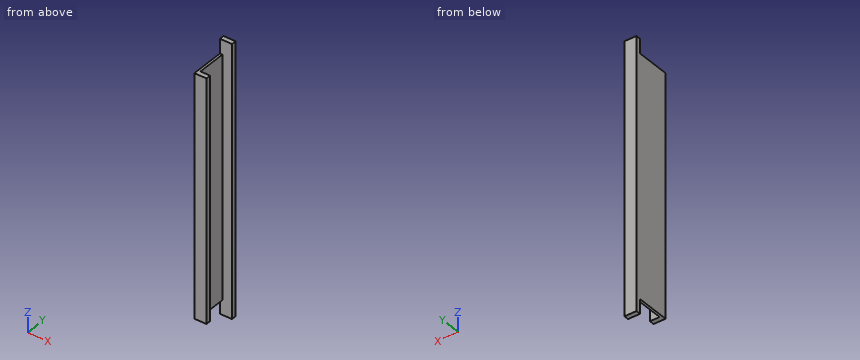
from build123d import *

# Parameters (mm, degrees)
CROQUIS1_R                   = 2.5
SALIENTE_EXTRUIR1_DEPTH      = 1.25
SALIENTE_EXTRUIR4_DEPTH      = 2.5
CROQUIS6_R                   = 12.525
CORTAR_EXTRUIR3_DEPTH        = 10
SALIENTE_EXTRUIR5_DEPTH      = 200
CROQUIS8_R                   = 12.525
SALIENTE_EXTRUIR6_DEPTH      = 21
CROQUIS10_W                  = 18.5
CROQUIS10_H                  = 25.138120499
CROQUIS10_W_2                = 2.5
CROQUIS10_H_2                = 4.861879501
CROQUIS10_H_3                = 5
CORTAR_EXTRUIR5_DEPTH        = 98
SALIENTE_EXTRUIR7_DEPTH      = 50
SALIENTE_EXTRUIR8_DEPTH      = 15
SALIENTE_EXTRUIR8_DEPTH_BACK = 265
CROQUIS15_W                  = 250
CROQUIS15_H                  = 5
CROQUIS15_W_2                = 280
SALIENTE_EXTRUIR9_DEPTH      = 7.5


with BuildPart() as part:
    # Croquis1 → Saliente-Extruir1 (new, symmetric)
    with BuildSketch(Plane(origin=(0, 0, 0), x_dir=(0, 0, -1), z_dir=(1, 0, 0))):
        with BuildLine():
            Line((125, -2.5), (-125, -2.5))
            Line((-125, -2.5), (-125, 2.5))
            Line((-125, 2.5), (-123, 2.5))
            Line((-123, 2.5), (-117, 17.5))
            ThreePointArc((-117, 17.5), (-110, 24.5), (-103, 17.5))
            Line((-103, 17.5), (-97, 2.5))
            Line((-97, 2.5), (125, 2.5))
            Line((125, 2.5), (125, -2.5))
        make_face()
        with Locations((-110, 17.5)):
            Circle(CROQUIS1_R, mode=Mode.SUBTRACT)
    extrude(amount=SALIENTE_EXTRUIR1_DEPTH, both=True)

    # Croquis5 → Saliente-Extruir4 (add, through all)
    with BuildSketch(Plane(origin=(1.25, 0, 0), x_dir=(0, 0, -1), z_dir=(1, 0, 0))):
        with BuildLine():
            ThreePointArc((-100, 10), (-110, 5), (-120, 10))
            Line((-120, 10), (-121.0552482, 7.361879501))
            ThreePointArc((-121.0552482, 7.361879501), (-110, 2.5), (-98.9447518, 7.361879501))
            Line((-98.9447518, 7.361879501), (-100, 10))
        make_face()
        with BuildLine():
            Line((-121.0552482, 7.361879501), (-120, 10))
            ThreePointArc((-120, 10), (-113.952847075, 29.358541226), (-97.5, 17.5))
            ThreePointArc((-97.5, 17.5), (-98.141458774, 13.547152925), (-100, 10))
            Line((-100, 10), (-98.9447518, 7.361879501))
            ThreePointArc((-98.9447518, 7.361879501), (-96.020931308, 12.060731804), (-95, 17.5))
            ThreePointArc((-95, 17.5), (-115.439268196, 31.479068692), (-121.0552482, 7.361879501))
        make_face()
    extrude(amount=-SALIENTE_EXTRUIR4_DEPTH)

    # Croquis6 → Cortar-Extruir3 (cut)
    with BuildSketch(Plane(origin=(1.25, 0, 0), x_dir=(0, 0, -1), z_dir=(1, 0, 0))):
        with Locations((-110, 17.5)):
            Circle(CROQUIS6_R)
    extrude(amount=-CORTAR_EXTRUIR3_DEPTH, mode=Mode.SUBTRACT)

    # Croquis7 → Saliente-Extruir5 (add)
    with BuildSketch(Plane(origin=(0, 0, -125), x_dir=(-1, 0, 0), z_dir=(0, 0, -1))):
        Polygon((3.75, 37.8), (3.75, -2.5), (1.25, -2.5), (1.25, 2.5), (1.25, 32.8), (-1.25, 32.8), (-1.25, 37.8), align=None)
    extrude(amount=-SALIENTE_EXTRUIR5_DEPTH)

    # Croquis8 → Saliente-Extruir6 (add)
    with BuildSketch(Plane.ZY.offset(1.25)):
        with BuildLine():
            Line((98.9447518, 7.361879501), (97, 2.5))
            Line((97, 2.5), (95, 2.5))
            Line((95, 2.5), (95, -2.5))
            Line((95, -2.5), (125, -2.5))
            Line((125, -2.5), (125, 2.5))
            Line((125, 2.5), (123, 2.5))
            Line((123, 2.5), (121.0552482, 7.361879501))
            ThreePointArc((121.0552482, 7.361879501), (110, 32.5), (98.9447518, 7.361879501))
        make_face()
        with Locations(Location((110, 17.5, 0), (0, 0, 180))):
            Circle(CROQUIS8_R, mode=Mode.SUBTRACT)
    extrude(amount=SALIENTE_EXTRUIR6_DEPTH)

    # Croquis10 → Cortar-Extruir5 (cut)
    with BuildSketch(Plane.XY.offset(75)):
        with Locations((-13, 19.930939751)):
            Rectangle(CROQUIS10_W, CROQUIS10_H)
        Polygon((1.25, 37.8), (-3.75, 37.8), (-3.75, 32.5), (-1.25, 32.5), (-1.25, 32.8), (1.25, 32.8), align=None)
        with Locations((0, 19.930939751)):
            Rectangle(CROQUIS10_W_2, CROQUIS10_H)
        with Locations((-2.5, 19.930939751)):
            Rectangle(CROQUIS10_W_2, CROQUIS10_H)
        with Locations((-13, 4.930939751)):
            Rectangle(CROQUIS10_W, CROQUIS10_H_2)
        with Locations((-2.5, 4.930939751)):
            Rectangle(CROQUIS10_W_2, CROQUIS10_H_2)
        with Locations((0, 4.930939751)):
            Rectangle(CROQUIS10_W_2, CROQUIS10_H_2)
        with Locations((-2.5, 0)):
            Rectangle(CROQUIS10_W_2, CROQUIS10_H_3)
        with Locations((-13, 0)):
            Rectangle(CROQUIS10_W, CROQUIS10_H_3)
        Rectangle(CROQUIS10_W_2, CROQUIS10_H_3)
    extrude(amount=CORTAR_EXTRUIR5_DEPTH, mode=Mode.SUBTRACT)

    # Croquis11 → Saliente-Extruir7 (add)
    with BuildSketch(Plane.XY.offset(75)):
        Polygon((-3.75, 37.8), (-3.75, -2.5), (1.25, -2.5), (1.25, 2.5), (-1.25, 2.5), (-1.25, 32.8), (1.25, 32.8), (1.25, 37.8), align=None)
    extrude(amount=SALIENTE_EXTRUIR7_DEPTH)

    # Croquis14 → Saliente-Extruir8 (add, two sides: drawn at the far end of the back side and taken through both)
    with BuildSketch(Plane.XY.offset(125).offset(-SALIENTE_EXTRUIR8_DEPTH_BACK)):
        Polygon((-1.25, 32.8), (1.25, 32.8), (1.25, 37.8), (-3.75, 37.8), (-3.75, 32.8), align=None)
    extrude(amount=SALIENTE_EXTRUIR8_DEPTH + SALIENTE_EXTRUIR8_DEPTH_BACK)

    # Croquis15 → Saliente-Extruir9 (add)
    with BuildSketch(Plane(origin=(1.25, 0, 0), x_dir=(0, 0, -1), z_dir=(1, 0, 0))):
        Rectangle(CROQUIS15_W, CROQUIS15_H)
        with Locations((0, 35.3)):
            Rectangle(CROQUIS15_W_2, CROQUIS15_H)
    extrude(amount=SALIENTE_EXTRUIR9_DEPTH)


solid = part.part
Input: part model. Units: mm. Frame: model coordinates. Give positions to 0.01 mm unless a question says otherwise; leave off trailing zeros. Loops run counter-clockwise (first coordinate to the right, second up) from the corner with the lowest first, then second, coordinate; pieces in that order, holes last. Notation, with made-up numbers: M -16.75,26.5 L 26.25,26.5 A21 ccw 26.25,58.5 Z; hole C 42.25,-12.75 d8. An arc over 180 degrees is marked long. Use one line per item in the form item = value.
1. Section query A-A, the plane x = 3. Return the cut outline in (y, z).
Numbers:
outline = M -2.5,-125 L 2.5,-125 L 2.5,125 L -2.5,125 Z; M 32.8,-140 L 37.8,-140 L 37.8,140 L 32.8,140 Z
2. Line query: L1, parallel to Y at x = -1, z = -93.5; L2, parallel to X at y = 14, z = -19.5; L3, parallel to Z at x = -1.5, y = 28. Output: solid intervals per line, ascending.
Numbers:
L1 = -2.5 to 2.5, 32.8 to 37.8
L2 = -3.75 to -1.25
L3 = -125 to 125
3. Section query C-C, the plane y = 27. Return the cut outline in (x, z).
Numbers:
outline = M -3.75,-125 L -1.25,-125 L -1.25,125 L -3.75,125 Z
4. Section query B-B, the plane z = 45. Return the cut outline in (x, y).
Numbers:
outline = M -3.75,-2.5 L 8.75,-2.5 L 8.75,2.5 L -1.25,2.5 L -1.25,32.8 L 8.75,32.8 L 8.75,37.8 L -3.75,37.8 Z
5. First-contact query: pin 1 (5 mm diameter, centred on y = 23, z = 34, fed in from +X); pin 2 (6 mm diameter, centred on x = 4, y = 9, fed in from +Z). Flat tips, straight axial feed; report the tip coordinate or a pass-through.
Numbers:
pin_1 = -1.25
pin_2 = through
